from build123d import *

# Parameters (mm, degrees)
SKETCH1_R                      = 42
BOSS_EXTRUDE1_DEPTH            = 60
CUT_EXTRUDE1_REACH             = 47
CUT_EXTRUDE1_DIRECTION_2_REACH = 47


with BuildPart() as part:
    # Sketch1 → Boss-Extrude1 (new body)
    with BuildSketch(Plane.XY):
        with BuildLine():
            ThreePointArc((2.5, 44.930501889), (15.285447634, 42.324403016), (26.785714286, 36.159722209))
            ThreePointArc((26.785714286, 36.159722209), (-12.910485027, -43.108228639), (-2.5, 44.930501889))
            Line((-2.5, 44.930501889), (-7.5, 52))
            Line((-7.5, 52), (7.5, 52))
            Line((7.5, 52), (2.5, 44.930501889))
        make_face()
        Circle(SKETCH1_R, mode=Mode.SUBTRACT)
    extrude(amount=BOSS_EXTRUDE1_DEPTH)

    # Cut-Extrude1: up to this face of the body (flat: up to its plane)
    cut_extrude1_end = Plane(part.part.faces().sort_by_distance((5, 48.465250945, 30))[0])
    # Sketch2 → Cut-Extrude1 (cut, up to the picked face)
    with BuildSketch(Plane(origin=(0, 0, 0), x_dir=(0, 0, -1), z_dir=(1, 0, 0)), mode=Mode.PRIVATE) as cut_extrude1_sk1:
        Polygon((-60, 44.930501889), (-50.525141204, 52), (-60, 52), align=None)
    cut_extrude1_tool1 = split(extrude(cut_extrude1_sk1.sketch, amount=CUT_EXTRUDE1_REACH, mode=Mode.PRIVATE), bisect_by=cut_extrude1_end, keep=Keep.BOTH, mode=Mode.PRIVATE)
    add(cut_extrude1_tool1.solids().sort_by_distance((0, 49.643501, 56.841714))[0], mode=Mode.SUBTRACT)

    # Cut-Extrude1 direction 2: up to this face of the body (flat: up to its plane)
    cut_extrude1_direction_2_end = Plane(part.part.faces().sort_by_distance((-5, 48.465250945, 30))[0])
    # Sketch2 → Cut-Extrude1 direction 2 (cut, up to the picked face)
    with BuildSketch(Plane(origin=(0, 0, 0), x_dir=(0, 0, -1), z_dir=(1, 0, 0)), mode=Mode.PRIVATE) as cut_extrude1_direction_2_sk1:
        Polygon((-60, 44.930501889), (-50.525141204, 52), (-60, 52), align=None)
    cut_extrude1_direction_2_tool1 = split(extrude(cut_extrude1_direction_2_sk1.sketch, amount=-CUT_EXTRUDE1_DIRECTION_2_REACH, mode=Mode.PRIVATE), bisect_by=cut_extrude1_direction_2_end, keep=Keep.BOTH, mode=Mode.PRIVATE)
    add(cut_extrude1_direction_2_tool1.solids().sort_by_distance((0, 49.643501, 56.841714))[0], mode=Mode.SUBTRACT)


solid = part.part
Build history of the part. All positions in model axes, mm. A direction names the side the tool comes from. Round coordinates to 2 decimals unless told otherwise and drop trailing zeros. Write each loop counter-clockwise with the first axis right and the second up, starting at its lowest first coordinate (ties: lowest second). Pieces come first, ordered by that corner, then holes. Notation, with made-up numbers: (-6.75, 40) -> (42.25, 40) arc R35 ccw to (42.25, 72) -> close; hole circle Ø6 at (-39, 50). An arc over 180 degrees is marked (long way). Write item = value, one per line.
(1) Tool access for faces 4 (the face through (40.06, 12.62, 29.58)), 5 (the face through (-4.97, 48.42, 29.58)): list every direction of +Z, -Z, +X, -X, +Y, -Y with a clear straight run to the whole face (end or side of a thin tool).
Answer:
face_4 = +Z, -Z
face_5 = +Z, -Z, -X
(2) Flat gauge pins, fed straight in: pin 1 (1 mm diameter, centred on y = -14, z = 7.5, fed in from -X); pin 2 (2 mm diameter, centred on y = 4.5, z = 17, fed in from -X); pin 3 (8 mm diameter, centred on x = 20.5, z = 8, fed in from -Y). Where does each tip first touch, or does it go through?
Answer:
pin_1 = -42.93
pin_2 = -44.86
pin_3 = -41.87
(3) Probe L1, parallel to Y at x = 0, z = 37; L2, parallel to X at y = -23, z = 23; L3, parallel to Y at x = 27.5, z = 37.5. List the from-to ranges inside material, lowest first.
Answer:
L1 = -45 to -42, 42 to 52
L2 = -38.68 to -35.14, 35.14 to 38.68
L3 = -35.62 to -31.75, 31.75 to 35.62
(4) Band-saw the part on B-B (x = 0). Give the cut face in (y, z).
Answer:
outline = (-45, 0) -> (-42, 0) -> (-42, 60) -> (-45, 60) -> close; (42, 0) -> (52, 0) -> (52, 50.53) -> (44.93, 60) -> (42, 60) -> close
(5) Band-saw the part on C-C (z = 15). Give the cut face in (x, y).
Answer:
outline = (-7.5, 52) -> (-2.5, 44.93) arc R45 ccw (long way) to (2.5, 44.93) -> (7.5, 52) -> close; hole circle Ø84 at (0, 0)
(6) Band-saw the part on D-D (x = 11.5). Give the cut face in (y, z), then the cut area to 3 significant figures.
Answer:
outline = (-43.51, 0) -> (-40.39, 0) -> (-40.39, 60) -> (-43.51, 60) -> close; (40.39, 0) -> (43.51, 0) -> (43.51, 60) -> (40.39, 60) -> close
area = 373 mm2
(7) Two-plate mould, pull along Y, no slides. Class faces 1 (the face through (26.9, 32.5, 0)), 2 (the face through (5.035, 48.515, 29.58)), 3 (the face through (0, 52, 25)): pulls with the +Y half, pulls with the -Y half, needs draft (parallel to the pull), parting line crosses it, or undercut.
Answer:
face_1 = needs draft
face_2 = undercut
face_3 = pulls with the +Y half
(8) Band-saw the part on A-A (y = 0). Give the cut face in (x, z).
Answer:
outline = (-45, 0) -> (-42, 0) -> (-42, 60) -> (-45, 60) -> close; (42, 0) -> (45, 0) -> (45, 60) -> (42, 60) -> close
